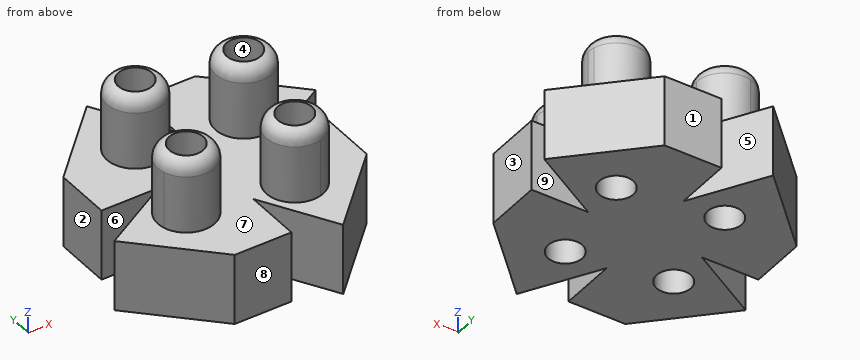
```python
from build123d import *

# Parameters (mm, degrees)
F1_DEPTH = 25
F2_DEPTH = 50
F3_R     = 6
F4_DEPTH = 50
F5_DEPTH = 50


# Not quite as in the source:
# - a fillet or chamfer that OpenCascade refuses, or shapes differently, is made with other operations: its cross-section is extruded or revolved along the edge and cut away or added


with BuildPart() as f1:
    # F0 (on Top) → F1 (new body)
    with BuildSketch(Plane.XY):
        Polygon((0, -20), (0, 0), (-20, 0), (-45.3589838486, -14.6410161514), (-20, -40), (0, -40), align=None)
        with BuildLine():
            ThreePointArc((-10, -14.6410161514), (-18.6986197214, -24.5559750202), (-29.6612818741, -17.2216425383))
            ThreePointArc((-29.6612818741, -17.2216425383), (-21.3013802786, -4.7260572825), (-10, -14.6410161514))
        make_face(mode=Mode.SUBTRACT)
        Polygon((-20, 0), (0, 0), (0, 20), (-14.6410161514, 45.3589838486), (-40, 20), (-40, 0), align=None)
        with BuildLine():
            ThreePointArc((-4.6410161514, 20), (-20.7317359828, 12.0688505288), (-17.2216425383, 29.6612818741))
            ThreePointArc((-17.2216425383, 29.6612818741), (-8.5502963199, 27.9311494712), (-4.6410161514, 20))
        make_face(mode=Mode.SUBTRACT)
        Polygon((0, 20), (0, 0), (20, 0), (45.3589838486, 14.6410161514), (20, 40), (0, 40), align=None)
        with BuildLine():
            ThreePointArc((30, 14.6410161514), (10.0850411312, 13.3396358728), (29.6612818741, 17.2216425383))
            ThreePointArc((29.6612818741, 17.2216425383), (29.9149588688, 15.9423964299), (30, 14.6410161514))
        make_face(mode=Mode.SUBTRACT)
        Polygon((20, 0), (0, 0), (0, -20), (14.6410161514, -45.3589838486), (40, -20), (40, 0), align=None)
        with BuildLine():
            ThreePointArc((24.6410161514, -20), (22.5721656226, -26.0907198315), (17.2216425383, -29.6612818741))
            ThreePointArc((17.2216425383, -29.6612818741), (6.7098666802, -13.9092801685), (24.6410161514, -20))
        make_face(mode=Mode.SUBTRACT)
        with BuildLine():
            ThreePointArc((-10, -14.6410161514), (-21.3013802786, -4.7260572825), (-29.6612818741, -17.2216425383))
            ThreePointArc((-29.6612818741, -17.2216425383), (-18.6986197214, -24.5559750202), (-10, -14.6410161514))
        make_face()
        with BuildLine():
            ThreePointArc((-4.6410161514, 20), (-8.5502963199, 27.9311494712), (-17.2216425383, 29.6612818741))
            ThreePointArc((-17.2216425383, 29.6612818741), (-20.7317359828, 12.0688505288), (-4.6410161514, 20))
        make_face()
        with BuildLine():
            ThreePointArc((30, 14.6410161514), (29.9149588688, 15.9423964299), (29.6612818741, 17.2216425383))
            ThreePointArc((29.6612818741, 17.2216425383), (10.0850411312, 13.3396358728), (30, 14.6410161514))
        make_face()
        with BuildLine():
            ThreePointArc((24.6410161514, -20), (6.7098666802, -13.9092801685), (17.2216425383, -29.6612818741))
            ThreePointArc((17.2216425383, -29.6612818741), (22.5721656226, -26.0907198315), (24.6410161514, -20))
        make_face()
    extrude(amount=F1_DEPTH)

    # F0 (on Top) → F2 (join)
    with BuildSketch(Plane.XY):
        with BuildLine():
            ThreePointArc((24.6410161514, -20), (6.7098666802, -13.9092801685), (17.2216425383, -29.6612818741))
            ThreePointArc((17.2216425383, -29.6612818741), (22.5721656226, -26.0907198315), (24.6410161514, -20))
        make_face()
        with BuildLine():
            ThreePointArc((-10, -14.6410161514), (-21.3013802786, -4.7260572825), (-29.6612818741, -17.2216425383))
            ThreePointArc((-29.6612818741, -17.2216425383), (-18.6986197214, -24.5559750202), (-10, -14.6410161514))
        make_face()
        with BuildLine():
            ThreePointArc((-4.6410161514, 20), (-8.5502963199, 27.9311494712), (-17.2216425383, 29.6612818741))
            ThreePointArc((-17.2216425383, 29.6612818741), (-20.7317359828, 12.0688505288), (-4.6410161514, 20))
        make_face()
        with BuildLine():
            ThreePointArc((30, 14.6410161514), (29.9149588688, 15.9423964299), (29.6612818741, 17.2216425383))
            ThreePointArc((29.6612818741, 17.2216425383), (10.0850411312, 13.3396358728), (30, 14.6410161514))
        make_face()
    extrude(amount=F2_DEPTH)

    # F3 (on face) → F4 (cut)
    with BuildSketch(Plane.XY.offset(50)):
        with Locations((-14.6410161514, 20)):
            Circle(F3_R)
    extrude(amount=-F4_DEPTH, mode=Mode.SUBTRACT)

    # F3 (on face) → F5 (cut)
    with BuildSketch(Plane.XY.offset(50)):
        with Locations((20, 14.6410161514)):
            Circle(F3_R)
        with Locations((14.6410161514, -20)):
            Circle(F3_R)
        with Locations((-20, -14.6410161514)):
            Circle(F3_R)
        with Locations((-14.6410161514, 20)):
            Circle(F3_R)
    extrude(amount=-F5_DEPTH, mode=Mode.SUBTRACT)

    # F6: fillet of radius 5 on 4 edges, made by hand

    # F6_s1 → F6_t2 (revolve, cut)
    with BuildSketch(Plane.XZ.offset(14.6410161514)):
        with BuildLine():
            ThreePointArc((-10, 45.1010205144), (-11.1270166538, 48.2632981746), (-14, 50))
            Line((-14, 50), (-10, 50))
            Line((-10, 50), (-10, 45.1010205144))
        make_face()
    revolve(axis=Axis((-20, -14.6410161514, 50), (0, 0, 1)), mode=Mode.SUBTRACT)

    # F6_s3 → F6_t4 (revolve, cut)
    with BuildSketch(Plane.XZ.offset(-20)):
        with BuildLine():
            ThreePointArc((-4.6410161514, 45.1010205144), (-5.7680328052, 48.2632981746), (-8.6410161514, 50))
            Line((-8.6410161514, 50), (-4.6410161514, 50))
            Line((-4.6410161514, 50), (-4.6410161514, 45.1010205144))
        make_face()
    revolve(axis=Axis((-14.6410161514, 20, 50), (0, 0, 1)), mode=Mode.SUBTRACT)

    # F6_s5 → F6_t6 (revolve, cut)
    with BuildSketch(Plane(origin=(8.6795464871, 2.3183949069, 0), x_dir=(0, 0, 1), z_dir=(-0.9661281874, -0.2580626387, 0))):
        with BuildLine():
            ThreePointArc((45.1010205144, -33.1008630094), (48.2632981746, -31.9738463556), (50, -29.1008630094))
            Line((50, -29.1008630094), (50, -33.1008630094))
            Line((50, -33.1008630094), (45.1010205144, -33.1008630094))
        make_face()
    revolve(axis=Axis((14.6410161514, -20, 50), (0, 0, 1)), mode=Mode.SUBTRACT)

    # F6_s7 → F6_t8 (revolve, cut)
    with BuildSketch(Plane.XZ.offset(-14.6410161514)):
        with BuildLine():
            ThreePointArc((30, 45.1010205144), (28.8729833462, 48.2632981746), (26, 50))
            Line((26, 50), (30, 50))
            Line((30, 50), (30, 45.1010205144))
        make_face()
    revolve(axis=Axis((20, 14.6410161514, 50), (0, 0, 1)), mode=Mode.SUBTRACT)


solid = f1.part
```
Design review of the part built by this model. Coordinates are the model's own, in mm. Face numbers are marked on the shaded views. A direction names the side the tool comes from. Coordinates: 2 decimals unless noted, no trailing zeros. Write each loop counter-clockwise with the first axis right and the second up, starting at its lowest first coordinate (ties: lowest second). Pieces come first, ordered by that corner, then holes.
1) To check wall thickness, follow L1, parallel to Y at x = 20, z = 29.5; L2, parallel to Y at x = 25, z = 15; L3, parallel to X at y = 21.5, z = 17. State the ranges of each line that lie inside material, in increasing order.
2) Add section B-B (z = 21). Write out the cut boundary in (x, y), plus the area to 3 significant figures.
3) Insertion check: pin 1 (12 mm diameter, centred on y = 30, z = 12, fed in from +X); pin 2 (6 mm diameter, centred on x = 7.5, z = 42.5, fed in from -Y); pin 3 (1.5 mm diameter, centred on y = -31, z = 9.5, fed in from -X); pin 4 (9.5 mm diameter, centred on x = 20, y = 14.64, fed in from -Z). Each pin has a flat end and moves straight along its axis. Give the tip position at first contact, or say it passes through.
4) Machinability: for the marked faces 5, 6, 7, 8 and 9, which of the approach directions +Z, -Z, +X, -X, +Y, -Y give a long, thin tool a straight path to every point of the face, cutting with its end or side? Answer none if there is none.
5) Mouldability with a two-part tool opening along X and no side actions: class the marked faces 1, 2, 3 and 4 as +X half, -X half, draft (parallel to the pull), parting line (faces both ways), or undercut.
6) Add section D-D (y = -34). Write out the cut boundary in (x, z).
7) Add section A-A (z = 26.5). Write out the cut boundary in (x, y).
8) Add section C-C (x = -34). Write out the cut boundary in (y, z).
Check result:
1. L1: y = -28.44 to -22.7, -17.3 to -11.56, 4.64 to 8.64, 20.64 to 24.64
1. L2: y = -35 to 0, 2.89 to 11.32, 17.96 to 35
1. L3: x = -38.5 to -20.45, -8.83 to -0.87, 0 to 38.5
2. outline: (-45.36, -14.64) - (-20, -40) - (0, -40) - (0, -20) - (14.64, -45.36) - (40, -20) - (40, 0) - (20, 0) - (45.36, 14.64) - (20, 40) - (0, 40) - (0, 20) - (-14.64, 45.36) - (-40, 20) - (-40, 0) - (-20, 0) - close; hole circle Ø12 at (-20, -14.64); hole circle Ø12 at (-14.64, 20); hole circle Ø12 at (14.64, -20); hole circle Ø12 at (20, 14.64)
2. area: 4,780 mm2
3. pin 1: stops at x = 36
3. pin 2: stops at y = -29.1
3. pin 3: stops at x = -29.75
3. pin 4: passes through
4. face 5: +Z, -Z, +Y
4. face 6: +Z, -Z, -X
4. face 7: +Z
4. face 8: +Z, -Z, -X, -Y
4. face 9: +Z, -Z, +X
5. face 1: draft
5. face 2: -X half
5. face 3: +X half
5. face 4: undercut
6. outline: (-26, 0) - (0, 0) - (0, 25) - (-26, 25) - close; (8.08, 0) - (26, 0) - (26, 25) - (8.08, 25) - close
7. outline: circle Ø20 at (-20, -14.64); circle Ø20 at (-14.64, 20); circle Ø20 at (14.64, -20); circle Ø20 at (20, 14.64); hole circle Ø12 at (-20, -14.64); hole circle Ø12 at (-14.64, 20); hole circle Ø12 at (14.64, -20); hole circle Ø12 at (20, 14.64)
8. outline: (-26, 0) - (-8.08, 0) - (-8.08, 25) - (-26, 25) - close; (0, 0) - (26, 0) - (26, 25) - (0, 25) - close
